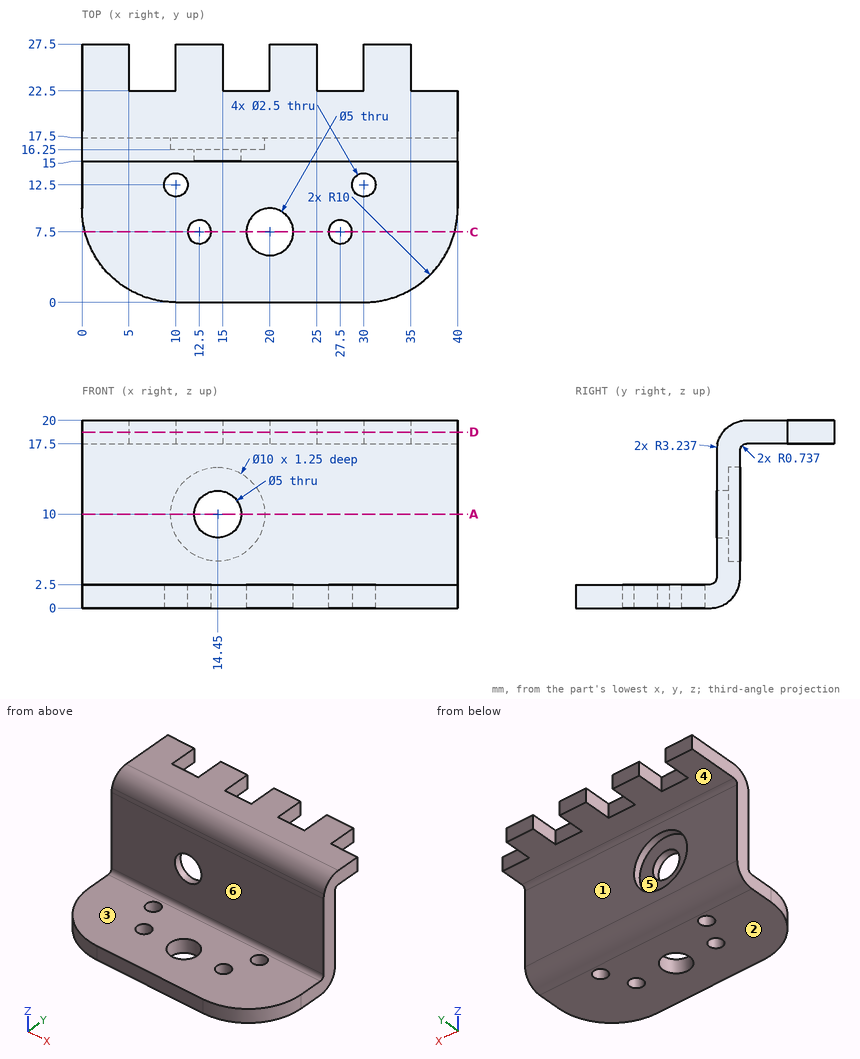
Could you check a few things on this drawing? It's one solid part, dimensions in mm from its lowest x, y, z. A direction names the side the tool comes from. Coordinates: 2 decimals unless noted, no trailing zeros. Order: outer loops, then holes, each group sorted by start corner. A loop starts at its lowest first (then second) coordinate and runs counter-clockwise, first axis right, second up.
1) Which directions (+Z, -Z, +X, -X, +Y, -Y) give clear straight access to the entire face, cutting with the end or side of a thin tool? Please do the marked faces 1, 2 and 3.
2) Will these pins go through, and if not, where does the flat tip stop? pin 1 (12 mm diameter, centred on y = 18.5, z = 4.5, fed in from -X); pin 2 (7 mm diameter, centred on x = 18, z = 8, fed in from -Y); pin 3 (7 mm diameter, centred on x = 11.5, z = 8, fed in from +Y); pin 4 (1.2 mm diameter, centred on y = 26, z = 18.5, fed in from +X).
3) Imagine slicing it at D-D on z = 18.75. List the corners of the cut face in (x, y) for me, and give its area (3 significant figures).
4) I need wall thicknesses on line 1 (Z direction, x = 6.5, y = 10.25); line 2 (Y direction, x = 26, z = 15.5); line 3 (Y direction, x = 20, z = 0.8) (1 decimal). Which ranges of each line are inside material? Lowest first, please.
5) Imagine slicing it at A-A on z = 10. List the corners of the cut face in (x, y) for me.
6) Imagine slicing it at C-C on y = 7.5. List the corners of the cut face in (x, z) for me.
7) We'd pull the mould along Z, two halves only. Please class the marked faces 4, 5 and 6: +Z half, -Z half, draft (parallel to the pull), parting line (faces both ways), or undercut.
Response values:
1. face 1: -Z, +X, -X, +Y
1. face 2: -Z, +X, -X, +Y, -Y
1. face 3: +Z, +X, -X, -Y
2. pin 1: stops at x = 0
2. pin 2: stops at y = 15
2. pin 3: stops at y = 17.5
2. pin 4: stops at x = 35
3. outline: (0, 15.68) - (40, 15.68) - (40, 22.5) - (35, 22.5) - (35, 27.5) - (30, 27.5) - (30, 22.5) - (25, 22.5) - (25, 27.5) - (20, 27.5) - (20, 22.5) - (15, 22.5) - (15, 27.5) - (10, 27.5) - (10, 22.5) - (5, 22.5) - (5, 27.5) - (0, 27.5) - close
3. area: 373 mm2
4. line 1: z = 0 to 2.5
4. line 2: y = 15 to 17.5
4. line 3: y = 0 to 5, 10 to 16.4
5. outline: (0, 15) - (11.95, 15) - (11.95, 16.25) - (9.45, 16.25) - (9.45, 17.5) - (0, 17.5) - close; (16.95, 15) - (40, 15) - (40, 17.5) - (19.45, 17.5) - (19.45, 16.25) - (16.95, 16.25) - close
6. outline: (0.32, 0) - (11.25, 0) - (11.25, 2.5) - (0.32, 2.5) - close; (13.75, 0) - (17.5, 0) - (17.5, 2.5) - (13.75, 2.5) - close; (22.5, 0) - (26.25, 0) - (26.25, 2.5) - (22.5, 2.5) - close; (28.75, 0) - (39.68, 0) - (39.68, 2.5) - (28.75, 2.5) - close
7. face 4: -Z half
7. face 5: undercut
7. face 6: draft
